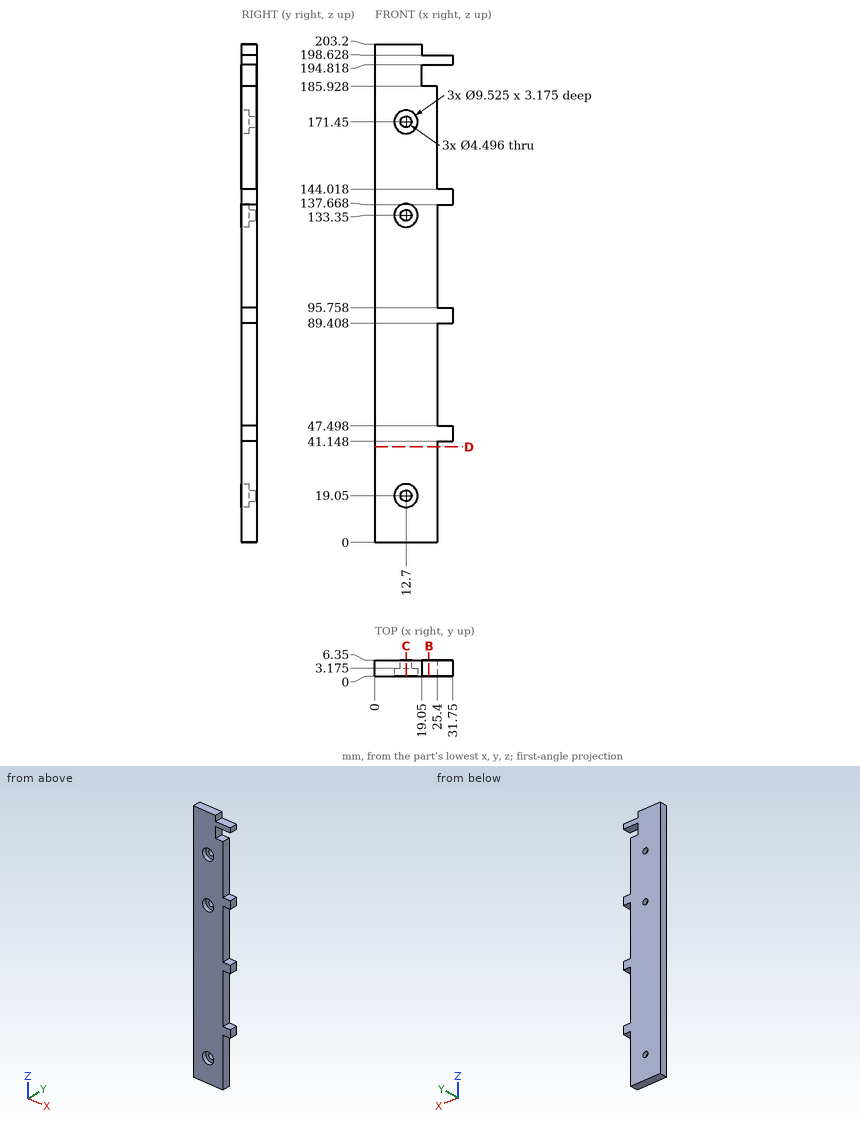
The figure shows three views and two pictorial views of one solid part (mm, origin at its lowest corner). Answer the questions. Give positions to 0.01 mm unless a question says otherwise; leave off trailing zeros. Loops run counter-clockwise (first coordinate to the right, second up) from the corner with the lowest first, then second, coordinate; pieces in that order, holes last. Notation, with made-up numbers: (30, -10.75) -> (51, -10.75) arc R21 cw to (51, 20.25) -> close; hole circle Ø7 at (14, 13). An arc over 180 degrees is marked (long way). Put each result on its own line as item: value. Start each with the question number.
Item 1: The part is cut by section D-D (z = 39). Give the vertices of the cut face in (x, y).
Item 2: Find the intervals of material crossed by L1, parallel to Z at x = 13, y = 2; L2, parallel to Z at x = 12.7, y = 4; L3, parallel to Z at x = 25, y = 3.75, in increasing order. Write a range as [from, to].
Item 3: The part is cut by section B-B (x = 22). Give the vertices of the cut face in (y, z), then the cut area to 4 significant figures.
Item 4: The part is cut by section C-C (x = 12.7). State how many separate pieces and enclosed holes the cut face has, then the cut area to 3 significant figures.
Item 5: Each of these flat-tipped pins is pushed along its axis until it touches: P1, Ø3, axis at y = 2, z = 81, coming from the +X side; P2, Ø2.5, axis at y = 4.5, z = 202, coming from the +X side; P3, Ø1.9, axis at x = 27, y = 3, coming from the +Z side. Where does it stop, or does it pass through?
Answers below:
1. outline: (0, 0) -> (25.4, 0) -> (25.4, 6.35) -> (0, 6.35) -> close
2. L1: [0, 14.3], [23.8, 128.6], [138.1, 166.7], [176.2, 203.2]
2. L2: [0, 16.8], [21.3, 131.1], [135.6, 169.2], [173.7, 203.2]
2. L3: [0, 185.93], [194.82, 198.63]
3. outline: (0, 0) -> (6.35, 0) -> (6.35, 185.93) -> (0, 185.93) -> close; (0, 194.82) -> (6.35, 194.82) -> (6.35, 198.63) -> (0, 198.63) -> close
3. area: 1,205 mm2
4. separate pieces: 4
4. enclosed holes: 0
4. area: 1,160 mm2
5. P1: x = 25.4
5. P2: x = 19.05
5. P3: z = 198.63
